For this review, take the finished solid that the model builds, in its own axes (mm). Give positions to 0.01 mm unless a question says otherwise; leave off trailing zeros. Loops run counter-clockwise (first coordinate to the right, second up) from the corner with the lowest first, then second, coordinate; pieces in that order, holes last.
```python
from build123d import *

# Parameters (mm, degrees)
F0_R     = 38.1
F1_DEPTH = 69.85
F2_R     = 28.575
F3_DEPTH = 25.4


# Not quite as in the source:
# - a fillet or chamfer that OpenCascade refuses, or shapes differently, is made with other operations: its cross-section is extruded or revolved along the edge and cut away or added


with BuildPart() as f1:
    # F0 (on Front) → F1 (new body)
    with BuildSketch(Plane.XZ):
        Circle(F0_R)
    extrude(amount=F1_DEPTH)

    # F2 (on face) → F3 (cut)
    with BuildSketch(Plane.XZ.offset(69.85)):
        Circle(F2_R)
    extrude(amount=-F3_DEPTH, mode=Mode.SUBTRACT)

    # F4: fillet of radius 28.59786 on 1 edges, made by hand

    # F4_s1 → F4_t2 (revolve)
    with BuildSketch(Plane.XY):
        with BuildLine():
            ThreePointArc((28.575, -69.85), (19.2141159123, -51.7254592304), (0.1564974356, -44.45))
            Line((0.1564974356, -44.45), (28.575, -44.45))
            Line((28.575, -44.45), (28.575, -69.85))
        make_face()
    revolve(axis=Axis((0, -44.45, 0), (0, -1, 0)))

    # F5: fillet of radius 22.86 on 1 edges, made by hand

    # F5_s1 → F5_t2 (revolve, cut)
    with BuildSketch(Plane.XY):
        with BuildLine():
            ThreePointArc((38.1, -51.2823567731), (35.5798340701, -61.7164714936), (28.575, -69.85))
            Line((28.575, -69.85), (38.1, -69.85))
            Line((38.1, -69.85), (38.1, -51.2823567731))
        make_face()
    revolve(axis=Axis((0, -69.85, 0), (0, -1, 0)), mode=Mode.SUBTRACT)


solid = f1.part
```
Q1. For pin 1 Ø2 at (x, z) = (-30, 19) entering from -Y; pin 2 Ø12 at (y, z) = (-53, -12) entering from +X; pin 3 Ø1 at (x, z) = (21.5, 9) entering from -Y, all flat-tipped, find the tip position at first contact; note any pin that passes through.
Answers:
pin 1: stops at y = -63.58
pin 2: stops at x = 37.6
pin 3: stops at y = -56.97
Q2. For probe 1 along Z at (x, y) = (-18.5, -61.5); probe 2 along Z at (x, y) = (23, -59.5); probe 3 along X at (y, z) = (-63, 5.5), list the stretches that pass through material, from the lowest coordinate up.
Answers:
probe 1: z = -30.52 to -18.72, 18.72 to 30.52
probe 2: z = -28.43 to -10.64, 10.64 to 28.43
probe 3: x = -34.43 to -26.36, 26.36 to 34.43
Q3. Consider section A-A on y = -18. Give the boundary of the cut face in (x, z), plus the area to 3 significant figures.
Answers:
outline: circle Ø76.2 at (0, 0)
area: 4,560 mm2
